```python
from build123d import *

# Parameters (mm, degrees)
F2_W     = 224
F2_H     = 135
F3_DEPTH = 10


with BuildPart() as f3:
    # F2 (on face) → F3 (new body)
    with BuildSketch(Plane(origin=(0, 0, 0), x_dir=(-1, 0, 0), z_dir=(0, 0.866025, -0.5))):
        with BuildLine():
            Line((-112, 188.748146), (-272, 188.748146))
            Line((-272, 188.748146), (-272, 95.748146))
            ThreePointArc((-272, 95.748146), (-269, 92.748146), (-272, 89.748146))
            Line((-272, 89.748146), (-282, 89.748146))
            Line((-282, 89.748146), (-282, 64.748146))
            Line((-282, 64.748146), (-272, 64.748146))
            ThreePointArc((-272, 64.748146), (-269, 61.748146), (-272, 58.748146))
            Line((-272, 58.748146), (-272, -34.251854))
            Line((-272, -34.251854), (-112, -34.251854))
            Line((-112, -34.251854), (48, -34.251854))
            Line((48, -34.251854), (48, 58.748146))
            ThreePointArc((48, 58.748146), (45, 61.748146), (48, 64.748146))
            Line((48, 64.748146), (58, 64.748146))
            Line((58, 64.748146), (58, 89.748146))
            Line((58, 89.748146), (48, 89.748146))
            ThreePointArc((48, 89.748146), (45, 92.748146), (48, 95.748146))
            Line((48, 95.748146), (48, 188.748146))
            Line((48, 188.748146), (-112, 188.748146))
        make_face()
        with Locations((-112, 77.248146)):
            Rectangle(F2_W, F2_H, mode=Mode.SUBTRACT)
    extrude(amount=F3_DEPTH)


solid = f3.part
```
The model under review builds one solid part; all positions refer to its coordinate system, in mm. A direction names the side the tool comes from. Coordinates: 2 decimals unless noted, no trailing zeros. Write each loop counter-clockwise with the first axis right and the second up, starting at its lowest first coordinate (ties: lowest second). Pieces come first, ordered by that corner, then holes.
1) To check wall thickness, follow probe 1 along Z at (x, y) = (104, 87.5); probe 2 along Z at (x, y) = (219, 90.5); probe 3 along Y at (x, z) = (185.5, -26). State the ranges of each line that lie inside material, in increasing order.
2) We need section C-C on x = -7. State the section outline as (y, z) points, then the cut area to 3 significant figures.
3) The part is to be moulded in two halves that separate along Z. For faces 6 (the face through (-52.93, 36.64, 53.61)), 7 (the face through (269, 35, 51)), 8 (the face through (272, 76, 121)), say which applies: pulls with the +Z half, pulls with the -Z half, needs draft (parallel to the pull), parting line crosses it, or undercut.
4) We need section A-A on x = 107. State the section outline as (y, z) points, then the cut area to 3 significant figures.
5) We need section B-B on y = 24. State the section outline as (x, z) points, then the cut area to 3 significant figures.
6) Machinability: for faces 1 (the face through (113.568, 76.644, 122.891)), 2 (the face through (113.6, 9.1, 6)), 3 (the face through (109.76, 98.64, 161)), 4 (the face through (277.07, 36.64, 53.61)), 5 (the face through (114.38, 85.232, 127.625)), which of the approach directions +Z, -Z, +X, -X, +Y, -Y give a long, thin tool a straight path to every point of the face, cutting with its end or side? Answer none if there is none.
7) We need section D-D on z = 139. State the section outline as (x, y) points.
8) Clearance check with flat-ended pins moving along their axes: pin 1 Ø1 at (x, z) = (229.5, 113) entering from +Y; pin 2 Ø12 at (x, z) = (174.5, 137.5) entering from +Y; pin 3 Ø3 at (x, z) = (107, 11) entering from -Y; pin 4 Ø16.5 at (y, z) = (23.5, 22.5) entering from +X. State where each tip first meets the part, or that it passes through.
Answer list:
1. probe 1: z = 131.55 to 151.55
1. probe 2: z = 136.75 to 156.75
1. probe 3: y = -15.01 to -3.46
2. outline: (-17.13, -29.66) - (-8.47, -34.66) - (103.03, 158.46) - (94.37, 163.46) - close
2. area: 2,230 mm2
3. face 6: pulls with the -Z half
3. face 7: undercut
3. face 8: needs draft
4. outline: (-17.13, -29.66) - (-8.47, -34.66) - (13.53, 3.44) - (4.87, 8.44) - close; (72.37, 125.36) - (81.03, 120.36) - (103.03, 158.46) - (94.37, 163.46) - close
4. area: 880 mm2
5. outline: (-48, 21.57) - (0, 21.57) - (0, 41.57) - (-48, 41.57) - close; (224, 21.57) - (272, 21.57) - (272, 41.57) - (224, 41.57) - close
5. area: 1,920 mm2
6. face 1: -Z, -Y
6. face 2: +Z, +Y
6. face 3: +Z, +X, -X, +Y
6. face 4: -Z, +X, -Y
6. face 5: -Z, +X, -X, +Y
7. outline: (-48, 80.25) - (272, 80.25) - (272, 91.8) - (-48, 91.8) - close
8. pin 1: stops at y = 77.08
8. pin 2: stops at y = 94.4
8. pin 3: passes through
8. pin 4: stops at x = 272
